```python
from build123d import *

# Parameters (mm, degrees)
BOSS_EXTRUDE1_START             = 0.2
SKETCH2_W                       = 41.966567091
SKETCH2_H                       = 11
SKETCH2_H_2                     = 34.4
SKETCH2_R                       = 4
SKETCH2_H_3                     = 4
BOSS_EXTRUDE1_DEPTH             = 4
BOSS_EXTRUDE2_REACH             = 197.713
SKETCH2_3_W                     = 41.966567091
SKETCH2_3_H                     = 11
SKETCH2_3_H_2                   = 4
BOSS_EXTRUDE2_DIRECTION_2_DEPTH = 60.2
FILLET1_R                       = 3
SKETCH3_W                       = 9
SKETCH3_H                       = 11.2
CUT_EXTRUDE1_DEPTH              = 24.029037182
SKETCH4_W                       = 71.659193782
SKETCH4_H                       = 19.690367256
SKETCH4_R                       = 3.18615952
BOSS_EXTRUDE3_DEPTH             = 4
FILLET2_R                       = 3
BOSS_EXTRUDE4_START             = -11
SKETCH5_W                       = 55.4
SKETCH5_H                       = 29.820392461
BOSS_EXTRUDE4_DEPTH             = 11
FILLET3_R                       = 3
CUT_EXTRUDE2_DEPTH              = 258.572392856
CUT_EXTRUDE2_DEPTH_BACK         = 258.572392856
SKETCH7_W                       = 8.5
SKETCH7_H                       = 4
FILLET6_R                       = 2
CUT_EXTRUDE3_REACH              = 172.81
CUT_EXTRUDE4_DEPTH              = 174.523300181
CUT_EXTRUDE4_DEPTH_BACK         = 174.523300181
FILLET7_R                       = 5
BOSS_EXTRUDE5_START             = -4
SKETCH10_W                      = 29.820392461
SKETCH10_H                      = 34.4
BOSS_EXTRUDE5_DEPTH             = 4
BOSS_EXTRUDE6_START             = 29.82039246
BOSS_EXTRUDE6_DEPTH             = 29.82039246
CUT_EXTRUDE5_DEPTH              = 210.306605099
CUT_EXTRUDE5_DEPTH_BACK         = 210.306605099
CUT_EXTRUDE6_DEPTH              = 210.306605099
CUT_EXTRUDE6_DEPTH_BACK         = 210.306605099
SKETCH15_W                      = 78.727492145
SKETCH15_H                      = 13.85710387
CUT_EXTRUDE8_REACH              = 163.596
SKETCH16_W                      = 13.433327452
SKETCH16_H                      = 52.832089958
FILLET8_R                       = 5


with BuildPart() as part:
    # Sketch2 → Boss-Extrude1 (new body)
    # profile 1 of 3: a face of its own
    with BuildSketch(Plane.ZY.offset(-93.4).offset(BOSS_EXTRUDE1_START)):
        with Locations((5.257762951, -150)):
            Rectangle(SKETCH2_W, SKETCH2_H)
    # profile 2 of 3: a face of its own
    with BuildSketch(Plane.ZY.offset(-93.4).offset(BOSS_EXTRUDE1_START)):
        with Locations((5.257762951, -172.7)):
            Rectangle(SKETCH2_W, SKETCH2_H_2)
        with Locations((5.257762951, -173.849326746)):
            Circle(SKETCH2_R, mode=Mode.SUBTRACT)
    # profile 3 of 3: a face of its own
    with BuildSketch(Plane.ZY.offset(-93.4).offset(BOSS_EXTRUDE1_START)):
        with Locations((5.257762951, -191.9)):
            Rectangle(SKETCH2_W, SKETCH2_H_3)
    extrude(amount=BOSS_EXTRUDE1_DEPTH)

    # Sketch2<3> → Boss-Extrude2 (add, up to next)
    with BuildSketch(Plane.ZY.offset(-93.4), mode=Mode.PRIVATE) as boss_extrude2_sk1:
        with Locations((5.257762951, -150)):
            Rectangle(SKETCH2_3_W, SKETCH2_3_H)
    boss_extrude2_tool1 = extrude(boss_extrude2_sk1.sketch, amount=BOSS_EXTRUDE2_REACH, mode=Mode.PRIVATE) - part.part
    # Sketch2<3> → Boss-Extrude2 (add, up to next)
    with BuildSketch(Plane.ZY.offset(-93.4), mode=Mode.PRIVATE) as boss_extrude2_sk2:
        with Locations((5.257762951, -191.9)):
            Rectangle(SKETCH2_3_W, SKETCH2_3_H_2)
    boss_extrude2_tool2 = extrude(boss_extrude2_sk2.sketch, amount=BOSS_EXTRUDE2_REACH, mode=Mode.PRIVATE) - part.part
    add(boss_extrude2_tool1.solids().sort_by_distance((93.4, -150, 5.257763))[0])
    add(boss_extrude2_tool2.solids().sort_by_distance((93.4, -191.9, 5.257763))[0])

    # Sketch2<3> → Boss-Extrude2 direction 2 (add)
    with BuildSketch(Plane.ZY.offset(-93.4)):
        with Locations((5.257762951, -150)):
            Rectangle(SKETCH2_3_W, SKETCH2_3_H)
        with Locations((5.257762951, -191.9)):
            Rectangle(SKETCH2_3_W, SKETCH2_3_H_2)
    extrude(amount=-BOSS_EXTRUDE2_DIRECTION_2_DEPTH)

    # Fillet1
    fillet1_edges = [part.edges().sort_by_distance(p)[0] for p in [
        (89.2, -193.9, 5.257762951),
        (93.2, -155.5, 5.257762951),
        (153.6, -191.9, 26.241046496),
        (93.2, -189.9, 5.257762951),
        (153.6, -191.9, -15.725520595),
    ]]
    fillet(fillet1_edges, radius=FILLET1_R)

    # Sketch3 → Cut-Extrude1 (cut)
    with BuildSketch(Plane.XY.offset(26.241046496)):
        with Locations((149.1, -150.1)):
            Rectangle(SKETCH3_W, SKETCH3_H)
    extrude(amount=-CUT_EXTRUDE1_DEPTH, mode=Mode.SUBTRACT)

    # Sketch4 → Boss-Extrude3 (add)
    with BuildSketch(Plane(origin=(153.6, 0, 0), x_dir=(0, 0, -1), z_dir=(1, 0, 0))):
        with Locations((-20.104076296, -145.654816372)):
            Rectangle(SKETCH4_W, SKETCH4_H)
        with Locations((-39.297424086, -145.700936153)):
            Circle(SKETCH4_R, mode=Mode.SUBTRACT)
        with Locations((-9.68615952, -145.700936153)):
            Circle(SKETCH4_R, mode=Mode.SUBTRACT)
    extrude(amount=-BOSS_EXTRUDE3_DEPTH)

    # Fillet2
    fillet2_edges = [part.edges().sort_by_distance(p)[0] for p in [
        (149.6, -144.5, -6.75675564),
        (151.6, -135.809632744, -15.725520595),
        (151.6, -135.809632744, 55.933673187),
    ]]
    fillet(fillet2_edges, radius=FILLET2_R)

    # Sketch5 → Boss-Extrude4 (add)
    with BuildSketch(Plane(origin=(0, -144.5, 0), x_dir=(1, 0, 0), z_dir=(0, 1, 0)).offset(BOSS_EXTRUDE4_START)):
        with Locations((116.9, -41.151242727)):
            Rectangle(SKETCH5_W, SKETCH5_H)
    extrude(amount=BOSS_EXTRUDE4_DEPTH)

    # Fillet3
    fillet3_edges = [part.edges().sort_by_distance(p)[0] for p in [
        (144.6, -150, 56.061438957),
        (89.2, -144.5, 20.167959181),
    ]]
    fillet(fillet3_edges, radius=FILLET3_R)

    # Sketch7 → Cut-Extrude2 (cut, two sides: drawn at the far end of the back side and taken through both)
    with BuildSketch(Plane(origin=(0, 0, -15.725520595), x_dir=(-1, 0, 0), z_dir=(0, 0, -1)).offset(-CUT_EXTRUDE2_DEPTH_BACK)):
        with Locations((-128.677790471, -153.5)):
            Rectangle(SKETCH7_W, SKETCH7_H)
        with Locations((-110.122209529, -153.5)):
            Rectangle(SKETCH7_W, SKETCH7_H)
    extrude(amount=CUT_EXTRUDE2_DEPTH + CUT_EXTRUDE2_DEPTH_BACK, mode=Mode.SUBTRACT)

    # Fillet6
    fillet6_edges = [part.edges().sort_by_distance(p)[0] for p in [
        (144.6, -150, 2.212009314),
    ]]
    fillet(fillet6_edges, radius=FILLET6_R)

    # Sketch8 → Cut-Extrude3 (cut, up to next)
    with BuildSketch(Plane(origin=(0, -144.5, 0), x_dir=(1, 0, 0), z_dir=(0, 1, 0)), mode=Mode.PRIVATE) as cut_extrude3_sk1:
        with BuildLine():
            Line((113.122209529, 2.172515143), (113.122209529, -42.508433505))
            ThreePointArc((113.122209529, -42.508433505), (110.122209529, -45.508433505), (107.122209529, -42.508433505))
            Line((107.122209529, -42.508433505), (107.122209529, 2.172515143))
            ThreePointArc((107.122209529, 2.172515143), (110.122209529, 5.172515143), (113.122209529, 2.172515143))
        make_face()
    cut_extrude3_tool1 = extrude(cut_extrude3_sk1.sketch, amount=-CUT_EXTRUDE3_REACH, mode=Mode.PRIVATE) & part.part
    # Sketch8 → Cut-Extrude3 (cut, up to next)
    with BuildSketch(Plane(origin=(0, -144.5, 0), x_dir=(1, 0, 0), z_dir=(0, 1, 0)), mode=Mode.PRIVATE) as cut_extrude3_sk2:
        with BuildLine():
            Line((125.677790471, 2.172515143), (125.677790471, -42.508433505))
            ThreePointArc((125.677790471, -42.508433505), (128.677790471, -45.508433505), (131.677790471, -42.508433505))
            Line((131.677790471, -42.508433505), (131.677790471, 2.172515143))
            ThreePointArc((131.677790471, 2.172515143), (128.677790471, 5.172515143), (125.677790471, 2.172515143))
        make_face()
    cut_extrude3_tool2 = extrude(cut_extrude3_sk2.sketch, amount=-CUT_EXTRUDE3_REACH, mode=Mode.PRIVATE) & part.part
    add(cut_extrude3_tool1.solids().sort_by_distance((110.12221, -144.5, 20.167959))[0], mode=Mode.SUBTRACT)
    add(cut_extrude3_tool2.solids().sort_by_distance((128.67779, -144.5, 20.167959))[0], mode=Mode.SUBTRACT)

    # Sketch9 → Cut-Extrude4 (cut, two sides: drawn at the far end of the back side and taken through both)
    with BuildSketch(Plane(origin=(0, -135.809632744, 0), x_dir=(1, 0, 0), z_dir=(0, 1, 0)).offset(-CUT_EXTRUDE4_DEPTH_BACK)):
        Polygon((144.6, 47.11572478), (144.6, -77.58184164), (185.54461202, -56.674351197), (190.182137353, 46.607841752), align=None)
    extrude(amount=CUT_EXTRUDE4_DEPTH + CUT_EXTRUDE4_DEPTH_BACK, mode=Mode.SUBTRACT)

    # Fillet7
    fillet7_edges = [part.edges().sort_by_distance(p)[0] for p in [
        (144.6, -150, -15.725520595),
    ]]
    fillet(fillet7_edges, radius=FILLET7_R)

    # Sketch10 → Boss-Extrude5 (add)
    with BuildSketch(Plane.ZY.offset(-89.2).offset(BOSS_EXTRUDE5_START)):
        with Locations((41.151242727, -172.7)):
            Rectangle(SKETCH10_W, SKETCH10_H)
    extrude(amount=BOSS_EXTRUDE5_DEPTH)

    # Sketch11 → Boss-Extrude6 (add)
    with BuildSketch(Plane.XY.offset(26.241046496).offset(BOSS_EXTRUDE6_START)):
        with BuildLine():
            Line((93.2, -155.5), (93.2, -158.5))
            ThreePointArc((93.2, -158.5), (94.078679656, -156.378679656), (96.2, -155.5))
            Line((96.2, -155.5), (93.2, -155.5))
        make_face()
    extrude(amount=-BOSS_EXTRUDE6_DEPTH)

    # Sketch14 → Cut-Extrude5 (cut, two sides: drawn at the far end of the back side and taken through both)
    with BuildSketch(Plane.ZY.offset(-89.2).offset(-CUT_EXTRUDE5_DEPTH_BACK)):
        with BuildLine():
            Line((9.257762951, -168.408548592), (9.257762951, -179.290104899))
            ThreePointArc((9.257762951, -179.290104899), (5.257762951, -183.290104899), (1.257762951, -179.290104899))
            Line((1.257762951, -179.290104899), (1.257762951, -168.408548592))
            ThreePointArc((1.257762951, -168.408548592), (5.257762951, -164.408548592), (9.257762951, -168.408548592))
        make_face()
    extrude(amount=CUT_EXTRUDE5_DEPTH + CUT_EXTRUDE5_DEPTH_BACK, mode=Mode.SUBTRACT)

    # Sketch15 → Cut-Extrude6 (cut, two sides: drawn at the far end of the back side and taken through both)
    with BuildSketch(Plane.ZY.offset(-89.2).offset(-CUT_EXTRUDE6_DEPTH_BACK)):
        with Locations((22.135388596, -196.828551935)):
            Rectangle(SKETCH15_W, SKETCH15_H)
    extrude(amount=CUT_EXTRUDE6_DEPTH + CUT_EXTRUDE6_DEPTH_BACK, mode=Mode.SUBTRACT)

    # Sketch16 → Cut-Extrude8 (cut, up to next)
    with BuildSketch(Plane.XZ.offset(189.9), mode=Mode.PRIVATE) as cut_extrude8_sk1:
        with Locations((99.916663726, 10.690524384)):
            Rectangle(SKETCH16_W, SKETCH16_H)
    cut_extrude8_tool1 = extrude(cut_extrude8_sk1.sketch, amount=-CUT_EXTRUDE8_REACH, mode=Mode.PRIVATE) & part.part
    add(cut_extrude8_tool1.solids().sort_by_distance((99.916664, -189.9, 10.690524))[0], mode=Mode.SUBTRACT)

    # Fillet8
    fillet8_edges = [part.edges().sort_by_distance(p)[0] for p in [
        (91.2, -189.9, 56.061438957),
        (91.2, -189.9, -15.725520595),
    ]]
    fillet(fillet8_edges, radius=FILLET8_R)


with BuildPart() as body_2:
    # Mirror1: mirrored copy
    add(part.part.mirror(Plane(origin=(144.6, -155.5, 56.061438957), x_dir=(1, 0, 0), z_dir=(0, 0, 1))))


solid = body_2.part
```
Geometry check sheet. Reference: the model listing, model coordinates, mm. A direction names the side the tool comes from. Round coordinates to 2 decimals unless told otherwise and drop trailing zeros. Loops run counter-clockwise (first coordinate to the right, second up) from the corner with the lowest first, then second, coordinate; pieces in that order, holes last. Notation, with made-up numbers: (63, 13) -> (103, 13) arc R12 ccw to (103, 35) -> close; hole circle Ø3 at (-17.75, -12.5). An arc over 180 degrees is marked (long way). Use a Markdown table: item, result.
(1) Mould release check, pull along X, two halves, no side actions. Record for faces 1 (the flat face through (109, -151, 56.061)), 2 (the cylindrical face through (128.612, -147.951, 66.615)), 3 (the cylindrical face through (143.74, -149.92, 56.96)): released by +X, released by -X, zero draft, split by the parting line, or undercut.
Calculated:
| item | result |
|---|---|
| face 1 | zero draft |
| face 2 | undercut |
| face 3 | released by +X |
(2) Sectioned sample at A-A (z = 108.5). Enter the section's corners in (x, y).
Calculated:
| item | result |
|---|---|
| outline | (89.2, -189.9) -> (93.2, -189.9) -> (93.2, -182.94) -> (89.2, -182.94) -> close; (89.2, -164.76) -> (93.2, -164.76) -> (93.2, -158.5) arc R3 cw to (96.2, -155.5) -> (105.87, -155.5) -> (105.87, -151.5) -> (107.12, -151.5) -> (107.12, -144.5) -> (92.2, -144.5) arc R3 ccw to (89.2, -147.5) -> close; (113.12, -151.5) -> (114.37, -151.5) -> (114.37, -155.5) -> (124.43, -155.5) -> (124.43, -151.5) -> (125.68, -151.5) -> (125.68, -144.5) -> (113.12, -144.5) -> close; (131.68, -151.5) -> (132.93, -151.5) -> (132.93, -155.5) -> (144.6, -155.5) -> (144.6, -144.5) -> (131.68, -144.5) -> close |
(3) Sectioned sample at B-B (x = 109). Enter the section's corners in (y, z), then the cut area to 3 significant figures.
Calculated:
| item | result |
|---|---|
| outline | (-151.5, 56.06) -> (-144.5, 56.06) -> (-144.5, 66.83) -> (-151.5, 66.83) -> close; (-151.5, 117.08) -> (-144.5, 117.08) -> (-144.5, 127.85) -> (-151.5, 127.85) -> close |
| area | 151 mm² |
(4) Go/stop test with flat-tipped pins: P1, Ø9.5, axis at x = 137.5, z = 89, coming from the -Y side; P2, Ø12, axis at y = -168.5, z = 74, coming from the +X side; P3, Ø4, axis at x = 108.5, z = 90.5, coming from the -Y side. Record where each tip stops, or that it passes through.
Calculated:
| item | result |
|---|---|
| P1 | y = -155.5 |
| P2 | x = 93.2 |
| P3 | y = -151.5 |
(5) Scan lines: probe 1 along X at (y, z) = (-149.5, 83); probe 2 along X at (y, z) = (-146.5, 84); probe 3 along Y at (x, z) = (124.5, 101.5). Record each from-to range of solid material in increasing order.
Calculated:
| item | result |
|---|---|
| probe 1 | 89.2 to 107.12, 113.12 to 125.68, 131.68 to 144.6 |
| probe 2 | 89.37 to 107.12, 113.12 to 125.68, 131.68 to 144.6 |
| probe 3 | -151.5 to -144.5 |
(6) Sectioned sample at C-C (z = 74.5). Enter the section's corners in (x, y).
Calculated:
| item | result |
|---|---|
| outline | (89.2, -189.9) -> (93.2, -189.9) -> (93.2, -158.5) arc R3 cw to (96.2, -155.5) -> (105.87, -155.5) -> (105.87, -151.5) -> (107.12, -151.5) -> (107.12, -144.5) -> (92.2, -144.5) arc R3 ccw to (89.2, -147.5) -> close; (113.12, -151.5) -> (114.37, -151.5) -> (114.37, -155.5) -> (124.43, -155.5) -> (124.43, -151.5) -> (125.68, -151.5) -> (125.68, -144.5) -> (113.12, -144.5) -> close; (131.68, -151.5) -> (132.93, -151.5) -> (132.93, -155.5) -> (144.6, -155.5) -> (144.6, -144.5) -> (131.68, -144.5) -> close |
(7) Set-up check for faces 4 (the flat face through (114, -151.5, 91)), 5 (the cylindrical face through (91.23, -164.41, 106.95)), 6 (the cylindrical face through (110.056, -147.951, 117.295)), 7 (the flat face through (119, -155.5, 92)): record each of +Z, -Z, +X, -X, +Y, -Y from which the full face is reachable in a straight line by a thin tool's end or side.
Calculated:
| item | result |
|---|---|
| face 4 | +Z, -Z, -Y |
| face 5 | +X, -X |
| face 6 | +Y, -Y |
| face 7 | +Z, -Z, +X, -Y |
(8) Sectioned sample at D-D (z = 118.5). Enter the section's corners in (x, y).
Calculated:
| item | result |
|---|---|
| outline | (89.2, -189.9) -> (93.2, -189.9) -> (93.2, -158.5) arc R3 cw to (96.2, -155.5) -> (105.87, -155.5) -> (105.87, -151.5) -> (114.37, -151.5) -> (114.37, -155.5) -> (124.43, -155.5) -> (124.43, -151.5) -> (132.93, -151.5) -> (132.93, -155.5) -> (144.6, -155.5) -> (144.6, -144.5) -> (92.2, -144.5) arc R3 ccw to (89.2, -147.5) -> close |
